Geometry: see drawing. Coordinates: mm, zero at the bounding-box minimum. A direction names the side the tool comes from. Coordinates: 2 decimals unless noted, no trailing zeros. Write each loop counter-clockwise with the first axis right and the second up, starting at its lowest first coordinate (ties: lowest second). Pieces come first, ordered by that corner, then holes. Notation, with made-up numbers: (15.5, 59.5) - (23.5, 59.5) arc R19 ccw to (23.5, 94.5) - close; hole circle Ø3 at (-35, -12.75). An arc over 180 degrees is marked (long way). One line per question, with ' | ' between items. Start each with the question number.
1) First-contact query: P1, Ø2, axis at y = 2, z = 2, coming from the +X side; P2, Ø2, axis at y = 6, z = 2.5, coming from the +X side; P3, Ø1, axis at y = 3, z = 4.5, coming from the -X side (1 decimal); P4, Ø1.6, axis at x = 5.5, y = 4, coming from the -Z side (1 decimal). Flat tips, straight axial feed; report the tip coordinate or a pass-through.
2) Line query: line 1 (X direction, y = 4.5, z = 2.5) (1 decimal); line 2 (Z direction, x = 8.5, y = 6.75); line 3 (Z direction, x = 4, y = 6.25) (1 decimal). Output: solid intervals per line, ascending.
3) Draft query along Y for the marked faces 3, 4 and 5. Return one class per face: released by +Y, released by -Y, zero draft, split by the parting line, or undercut.
4) Section query C-C on x = 5.5. Return loops of the section in (y, z) (1 decimal).
5) Section query B-B on z = 2.75. Return loops of the section in (x, y).
6) Reachability of the marked faces 1 and 2 from +Z, -Z, +X, -X, +Y, -Y: full face, straight path, thin tool, end or side. Return the list, or none.
7) Section query A-A on y = 7.25. Return loops of the section in (x, z) (1 decimal).
8) Section query D-D on z = 9. Return loops of the section in (x, y) (1 decimal).
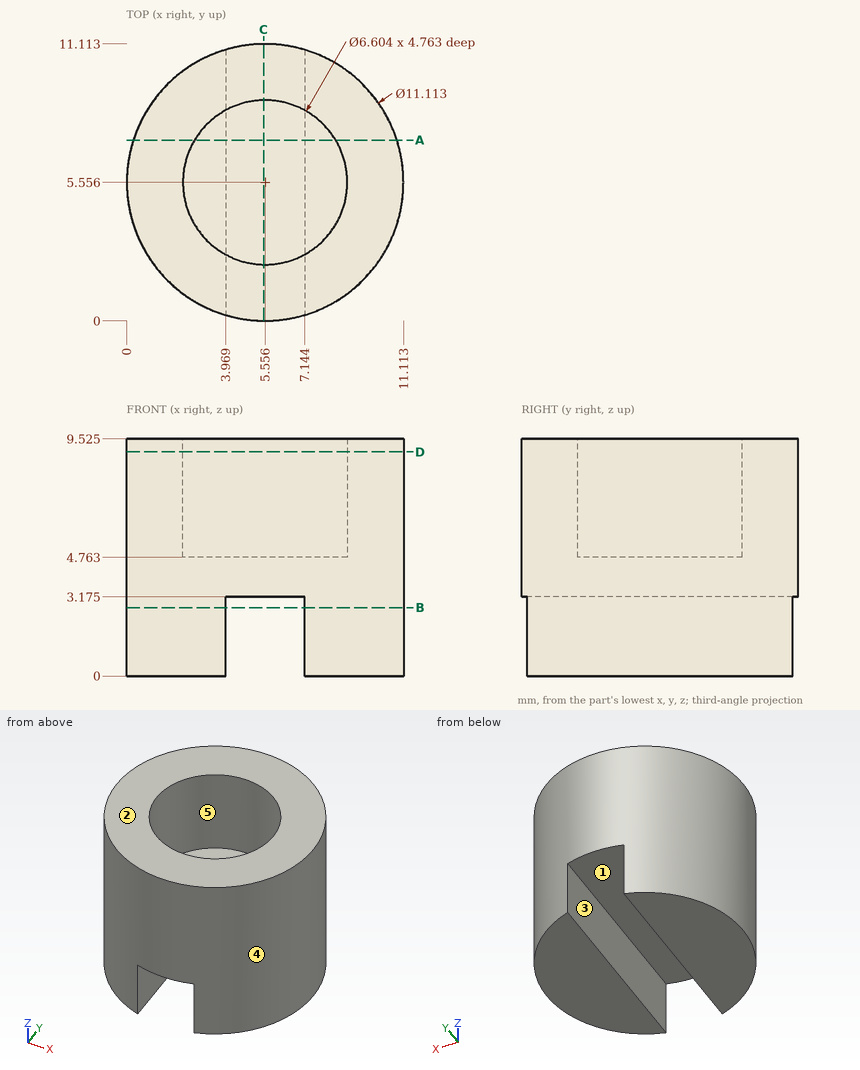
Answer key:
1) P1: x = 10.49 | P2: x = 11.11 | P3: x = 0.4 | P4: z = 3.2
2) line 1: 0.1 to 4, 7.1 to 11 | line 2: 0 to 4.76 | line 3: 3.2 to 4.8
3) face 3: zero draft | face 4: split by the parting line | face 5: undercut
4) outline: (0, 3.2) - (11.1, 3.2) - (11.1, 9.5) - (8.9, 9.5) - (8.9, 4.8) - (2.3, 4.8) - (2.3, 9.5) - (0, 9.5) - close
5) outline: (3.97, 0.23) - (3.97, 10.88) arc R5.56 ccw to start; (7.14, 0.23) arc R5.56 ccw to (7.14, 10.88) - close
6) face 1: -Z, +Y, -Y | face 2: +Z, +X, -X, +Y, -Y
7) outline: (0.3, 0) - (4, 0) - (4, 3.2) - (7.1, 3.2) - (7.1, 0) - (10.8, 0) - (10.8, 9.5) - (8.4, 9.5) - (8.4, 4.8) - (2.7, 4.8) - (2.7, 9.5) - (0.3, 9.5) - close
8) outline: circle Ø11.1 at (5.6, 5.6); hole circle Ø6.6 at (5.6, 5.6)
